Read the model definition and answer for the solid it produces. Units are mm, in the model's axes. A direction names the side the tool comes from. Round coordinates to 2 decimals unless told otherwise and drop trailing zeros. Order: outer loops, then holes, each group sorted by start corner. A loop starts at its lowest first (then second) coordinate and runs counter-clockwise, first axis right, second up. Notation, with made-up numbers: (12, 80.25) -> (40, 80.25) arc R29 cw to (40, 119.25) -> close; hole circle Ø7 at (37, 49.5). An arc over 180 degrees is marked (long way). One line per item, written item: value. Start each with the question number.
1. Section A-A (x = -18) is taken. Give the vertices of the cut face in (y, z), then the cut area to 3 significant figures.
2. Consider line 1 (Z direction, x = -11, y = 4.5); line 2 (X direction, y = 2.75, z = -11); line 3 (Z direction, x = -10, y = 7.5). Determine where each line is inside the solid, lowest interval first.
3. Section B-B (z = -68) is taken. Give the vertices of the cut face in (x, y).
4. Flat-ended cylindrical pins translate along their axes: pin 1 Ø1 at (y, z) = (5, -10.5) entering from -X; pin 2 Ø1.7 at (x, z) = (-29, -41) entering from -Y. Find the tip coordinate at first contact, or state that the pin passes through.
5. Section C-C (z = -41.7) is taken. Give the vertices of the cut face in (x, y) (3 decimals), then the cut area to 3 significant figures.
6. Section D-D (z = -10.35) is taken. State how many separate pieces and enclosed holes the cut face has, then the cut area to 3 significant figures.
7. For faces 1 (the face through (-29.34, 7.03, -40.19)), 2 (the face through (-31.51, 6.54, -47.25)), 3 (the face through (-21.9, 2.5, -44.1)), determine the directions among +Z, -Z, +X, -X, +Y, -Y from which every point of the face is accessible in a straight line to the end or side of a thin tool.
8. The mould has two halves that part along Y. Classify faces 4 (the face through (-33.24, 4.061, -8.957)), 5 (the face through (-8.6, 5, -26.21)), 6 (the face through (-21.203, 3, -9)): released by +Y, released by -Y, zero draft, split by the parting line, or undercut.
Autodesk Inventor part; units mm, degrees
ref_plane "Work Plane1" through (-30.1251, 9, -4) normal (1, 0, 0) x (0, 0, -1)
ref_plane "Work Plane2" through (-23.3752, 9, -4) normal (1, 0, 0) x (0, 0, -1)
ref_plane "Work Plane3" through (-30.1251, 9, -4) normal (1, 0, 0) x (0, 0, -1)
sketch "Sketch1" plane through (0, 0, 0) normal (0, 1, 0) x (-1, 0, 0)
  line L0 (0, 0) -> (35.5, 0)
  line L1 (35.5, 0) -> (35.5, -90)
  line L2 (35.5, -90) -> (0, -90)
  line L3 (0, -90) -> (0, 0)
  dimension "d0" = 35.5
  dimension "d1" = 90
extrude "Extrusion1" add sketch "Sketch1" along normal blind 9
sketch "Sketch2" plane through (0, 9, 0) normal (0, 1, 0) x (1, 0, 0)
  circle A0 centre (-10, 15) radius 3.25 construction
  line L0 (-35.5, 0) -> (0, 0)
  line L1 (0, 0) -> (0, 90)
  line L2 (-13.25, 15) -> (-11.625, 17.8146)
  line L3 (-11.625, 17.8146) -> (-8.375, 17.8146)
  line L4 (-8.375, 17.8146) -> (-6.75, 15)
  line L5 (-6.75, 15) -> (-8.375, 12.1854)
  line L6 (-8.375, 12.1854) -> (-11.625, 12.1854)
  line L7 (-11.625, 12.1854) -> (-13.25, 15)
  line L8 (0, 90) -> (-35.5, 90)
  circle A1 centre (-10, 15) radius 1.7 construction
  dimension "d7" = 6.5
  dimension "d24" = 15
  dimension "d25" = 10
  dimension "d28" = 3.4
extrude "Extrusion2" cut sketch "Sketch2" against normal blind 5
sketch "Sketch3" plane through (0, 0, 0) normal (0, -1, 0) x (1, 0, 0)
  circle A0 centre (-10, -25) radius 3.25 construction
  line L0 (0, 0) -> (-35.5, 0)
  line L1 (-35.5, 0) -> (-35.5, -90)
  line L2 (-11.6286, -27.8125) -> (-13.25, -24.9958)
  line L3 (-13.25, -24.9958) -> (-11.6214, -22.1833)
  line L4 (-11.6214, -22.1833) -> (-8.3714, -22.1875)
  line L5 (-8.3714, -22.1875) -> (-6.75, -25.0042)
  line L6 (-6.75, -25.0042) -> (-8.3786, -27.8167)
  line L7 (-8.3786, -27.8167) -> (-11.6286, -27.8125)
  line L8 (0, -90) -> (0, 0)
  dimension "d15" = 6.5
  dimension "d16" = 25
  dimension "d26" = 10
extrude "Extrusion3" cut sketch "Sketch3" against normal blind 5
sketch "Sketch5" plane through (0, 9, 0) normal (0, 1, 0) x (1, 0, 0)
  circle A0 centre (-10, 15) radius 1.7
  line L0 (0, 0) -> (0, 90)
  line L1 (-35.5, 0) -> (0, 0)
  circle A1 centre (-10, 25) radius 1.7
  dimension "d30" = 3.4
  dimension "d31" = 10
  dimension "d32" = 15
  dimension "d36" = 3.4
  dimension "d37" = 25
extrude "Extrusion4" cut sketch "Sketch5" against normal through all
sketch "Sketch6" plane through (0, 9, 0) normal (0, 1, 0) x (1, 0, 0)
  line L0 (-32.5, 4) -> (-27.7502, 4)
  line L1 (-27.7502, 4) -> (-27.7502, 16.7)
  line L2 (-27.7502, 16.7) -> (-32.5, 16.7)
  line L3 (-32.5, 16.7) -> (-32.5, 4)
  line L4 (-35.5, 0) -> (0, 0)
  line L5 (-35.5, 90) -> (-35.5, 0)
  line L6 (-25.7502, 4) -> (-21.0002, 4)
  line L7 (-21.0002, 4) -> (-21.0002, 16.7)
  line L8 (-21.0002, 16.7) -> (-25.7502, 16.7)
  line L9 (-25.7502, 16.7) -> (-25.7502, 4)
  line L10 (0, 0) -> (0, 90) construction
  line L11 (-35.5, 90) -> (0, 90)
  line L12 (0, 0) -> (-20, 0) construction
  line L13 (-20, 0) -> (-20, 90) construction
  line L14 (-20, 90) -> (0, 90) construction
  line L15 (0, 90) -> (0, 0)
  circle A0 centre (-23.3752, 41.7) radius 1.7
  circle A1 centre (-30.125, 41.7) radius 1.7
  circle A2 centre (-30.125, 49.7) radius 1.7
  circle A3 centre (-23.3752, 49.7) radius 1.7
  dimension "d43" = 4.7498
  dimension "d44" = 12.7
  dimension "d45" = 4
  dimension "d46" = 3
  dimension "d47" = 4.75
  dimension "d48" = 2
  dimension "d49" = 20
  dimension "d50" = 3.4
  dimension "d51" = 25
  dimension "d90" = 3.4
  dimension "d91" = 5.375
  dimension "d92" = 3.4
  dimension "d93" = 8
  dimension "d94" = 3.4
extrude "Extrusion5" cut sketch "Sketch6" against normal through all contours L3 L2 L1 L0 | L9 L8 L7 L6 | A0 | A1 | A2 | A3
sketch "Sketch7" plane through (0, 0, 0) normal (0, -1, 0) x (1, 0, 0)
  circle A0 centre (-23.3752, -41.7) radius 1.7
  circle A1 centre (-23.3752, -41.7) radius 3.25 construction
  line L0 (-23.3752, -38.45) -> (-20.5606, -40.075)
  line L1 (-20.5606, -40.075) -> (-20.5606, -43.325)
  line L2 (-20.5606, -43.325) -> (-23.3752, -44.95)
  line L3 (-23.3752, -44.95) -> (-26.1898, -43.325)
  line L4 (-26.1898, -43.325) -> (-26.1898, -40.075)
  line L5 (-26.1898, -40.075) -> (-23.3752, -38.45)
  line L6 (0, 0) -> (-35.5, 0)
  circle A2 centre (-30.125, -41.7) radius 3.25 construction
  line L7 (-35.5, 0) -> (-35.5, -90)
  line L8 (-30.1645, -44.9498) -> (-32.9591, -43.2907)
  line L9 (-32.9591, -43.2907) -> (-32.9196, -40.0409)
  line L10 (-32.9196, -40.0409) -> (-30.0855, -38.4502)
  line L11 (-30.0855, -38.4502) -> (-27.2909, -40.1093)
  line L12 (-27.2909, -40.1093) -> (-27.3304, -43.3591)
  line L13 (-27.3304, -43.3591) -> (-30.1645, -44.9498)
  dimension "d88" = 6.5
  dimension "d54" = 6.5
  dimension "d87" = 41.7
  dimension "d89" = 5.375
extrude "Extrusion6" cut sketch "Sketch7" against normal blind 5
sketch "Sketch8" plane through (-35.5, 0, -90) normal (-1, 0, 0) x (0, 0, 1)
  circle A0 centre (79.65, 4.5) radius 1.4605
  line L0 (0, 9) -> (90, 9)
  line L1 (90, 0) -> (90, 9)
  dimension "d57" = 2.921
  dimension "d58" = 4.5
  dimension "d59" = 10.35
hole "Hole1" at (-35.5, 4.5, -10.35) direction (1, 0, 0) diameter 2.921 depth 21 counterbore diameter 3.4 counterbore depth 1.5
sketch "Sketch9" plane through (-21.0002, 9, -16.7) normal (-1, 0, 0) x (0, 0, 1)
  circle A0 centre (6.35, -4.5) radius 1.4605
  circle A1 centre (6.35, -4.5) radius 2.54
  point P0 (16.7, -9)
  dimension "d67" = 5.08
extrude "Extrusion7" add sketch "Sketch9" along normal blind 0.2032
sketch "Sketch10" plane through (-27.7502, 9, -16.7) normal (-1, 0, 0) x (0, 0, 1)
  circle A0 centre (6.35, -4.5) radius 1.7
  circle A1 centre (6.35, -4.5) radius 2.54
  point P0 (16.7, -9)
  dimension "d70" = 5.08
extrude "Extrusion8" add sketch "Sketch10" along normal blind 0.2032
sketch "Sketch11" plane through (-25.7502, 9, -4) normal (1, 0, 0) x (0, 0, -1)
  circle A0 centre (6.35, -4.5) radius 1.7
  circle A1 centre (6.35, -4.5) radius 2.54
  point P0 (-4, -9)
  dimension "d73" = 5.08
extrude "Extrusion9" add sketch "Sketch11" along normal blind 0.2032
sketch "Sketch12" plane through (-32.5, 9, -4) normal (1, 0, 0) x (0, 0, -1)
  circle A0 centre (6.35, -4.5) radius 1.7
  circle A1 centre (6.35, -4.5) radius 2.54
  point P0 (-4, -9)
  dimension "d76" = 5.08
extrude "Extrusion10" add sketch "Sketch12" along normal blind 0.2032
sketch "Sketch14" plane through (0, 0, -90) normal (0, 0, -1) x (-1, 0, 0)
  circle A0 centre (18, 4.5) radius 2.25
  line L0 (35.5, 0) -> (0, 0)
  line L1 (0, 0) -> (0, 9)
  dimension "d82" = 4.5
  dimension "d83" = 4.5
  dimension "d84" = 18
extrude "Extrusion11" cut sketch "Sketch14" against normal blind 41
sketch "Sketch15" plane through (0, 9, 0) normal (0, 1, 0) x (1, 0, 0)
  circle A0 centre (-30.125, 49.7) radius 1.7
  circle A1 centre (-30.125, 49.7) radius 3.25 construction
  circle A2 centre (-23.3752, 49.7) radius 1.7
  circle A3 centre (-23.3752, 49.7) radius 3.25 construction
  line L0 (-30.125, 52.95) -> (-27.3104, 51.325)
  line L1 (-27.3104, 51.325) -> (-27.3104, 48.075)
  line L2 (-27.3104, 48.075) -> (-30.125, 46.45)
  line L3 (-30.125, 46.45) -> (-32.9396, 48.075)
  line L4 (-32.9396, 48.075) -> (-32.9396, 51.325)
  line L5 (-32.9396, 51.325) -> (-30.125, 52.95)
  line L6 (-23.3752, 52.95) -> (-20.5606, 51.325)
  line L7 (-20.5606, 51.325) -> (-20.5606, 48.075)
  line L8 (-20.5606, 48.075) -> (-23.3752, 46.45)
  line L9 (-23.3752, 46.45) -> (-26.1898, 48.075)
  line L10 (-26.1898, 48.075) -> (-26.1898, 51.325)
  line L11 (-26.1898, 51.325) -> (-23.3752, 52.95)
  point P0 (0, 0)
  dimension "d95" = 6.5
  dimension "d96" = 6.5
extrude "Extrusion12" cut sketch "Sketch15" against normal blind 5
ref_plane "Work Plane1" through (-30.1251, 9, -4) normal (1, 0, 0) x (0, 0, -1)
ref_plane "Work Plane2" through (-23.3752, 9, -4) normal (1, 0, 0) x (0, 0, -1)
ref_plane "Work Plane3" through (-30.1251, 9, -4) normal (1, 0, 0) x (0, 0, -1)
ref_plane "Work Plane4" through (-23.3752, 9, -4) normal (1, 0, 0) x (0, 0, -1)
properties part number "Bottom coupler"
Answer:
1. outline: (0, -90) -> (2.25, -90) -> (2.25, -49) -> (6.75, -49) -> (6.75, -90) -> (9, -90) -> (9, 0) -> (0, 0) -> close; hole circle Ø2.92 at (4.5, -10.35)
1. area: 619 mm^2
2. line 1: -90 to -27.81, -22.18 to -17.81, -12.19 to 0
2. line 2: -35.5 to -32.3, -27.95 to -25.55, -21.2 to 0
2. line 3: -90 to -26.7, -23.3 to -17.81, -12.19 to 0
3. outline: (-35.5, 0) -> (0, 0) -> (0, 9) -> (-35.5, 9) -> close; hole circle Ø4.5 at (-18, 4.5)
4. pin 1: x = -14.5
4. pin 2: y = 5
5. outline: (-35.5, 0) -> (-32.94, 0) -> (-32.94, 5) -> (-31.825, 5) -> (-31.825, 9) -> (-35.5, 9) -> close; (-28.425, 5) -> (-27.31, 5) -> (-27.31, 0) -> (-26.19, 0) -> (-26.19, 5) -> (-25.075, 5) -> (-25.075, 9) -> (-28.425, 9) -> close; (-21.675, 5) -> (-20.561, 5) -> (-20.561, 0) -> (0, 0) -> (0, 9) -> (-21.675, 9) -> close
5. area: 236 mm^2
6. separate pieces: 5
6. enclosed holes: 0
6. area: 201 mm^2
7. face 1: +Y, -Y
7. face 2: +Y
7. face 3: -Y
8. face 4: undercut
8. face 5: released by -Y
8. face 6: zero draft
